from build123d import *

# Parameters (mm, degrees)
F0_R     = 1.778
F1_DEPTH = 6.7564
F3_R     = 1.1684
F4_DEPTH = 3.175
F5_R     = 1.143
F6_DEPTH = 3.175


with BuildPart() as f1:
    # F0 (on Top) → F1 (new body)
    with BuildSketch(Plane.XY):
        Circle(F0_R)
    extrude(amount=F1_DEPTH)

    # F3 (on face) → F4 (cut)
    with BuildSketch(Plane.XY.offset(6.7564)):
        Circle(F3_R)
    extrude(amount=F4_DEPTH, mode=Mode.SUBTRACT)

    # F5 (on face) → F6 (join)
    with BuildSketch(Plane(origin=(0, 0, 0), x_dir=(1, 0, 0), z_dir=(0, 0, -1))):
        Circle(F5_R)
    extrude(amount=F6_DEPTH)


solid = f1.part
The model under review builds one solid part; all positions refer to its coordinate system, in mm. A direction names the side the tool comes from. Round coordinates to 2 decimals unless told otherwise and drop trailing zeros. Loops run counter-clockwise (first coordinate to the right, second up) from the corner with the lowest first, then second, coordinate; pieces in that order, holes last. Notation, with made-up numbers: (-10.5, 56.25) -> (7.5, 56.25) arc R30 cw to (7.5, 83.25) -> close; hole circle Ø9 at (-37.5, -36.75). An arc over 180 degrees is marked (long way). Return JSON: item names as keys, results as strings.
(1) For pin 1 (1 mm diameter, centred on x = 0.5, z = -1, fed in from +Y); pin 2 (1.5 mm diameter, centred on y = 1, z = 3.5, fed in from -X); pin 3 (1 mm diameter, centred on y = -1.5, z = 4, fed in from +X), all flat-tipped, find the tip position at first contact; note any pin that passes through.
Solved:
{"pin 1": "y = 1.14", "pin 2": "x = -1.76", "pin 3": "x = 1.47"}
(2) Add section D-D on z = -0.5. Write out the cut boundary in (x, y).
Solved:
{"outline": "circle Ø2.29 at (0, 0)"}
(3) For line 1 (Z direction, x = 1.3, y = -0.3); line 2 (X direction, y = 0.4, z = 4.75); line 3 (X direction, y = -1.35, z = 6), list the stretches that pass through material, from the lowest coordinate up.
Solved:
{"line 1": "0 to 6.76", "line 2": "-1.73 to 1.73", "line 3": "-1.16 to 1.16"}
(4) Add section A-A on y = 0. Write out the cut boundary in (x, z) (3 decimals).
Solved:
{"outline": "(-1.778, 0) -> (-1.143, 0) -> (-1.143, -3.175) -> (1.143, -3.175) -> (1.143, 0) -> (1.778, 0) -> (1.778, 6.756) -> (-1.778, 6.756) -> close"}
(5) For faces 1 (the flat face through (-1, 1, 0)), 2 (the flat face through (0, 0, 6.756)), list the 3-axis set-ups (+Z, -Z, +X, -X, +Y, -Y) from which the entire face can be reached by the end or side of a thin tool; tool diameter is ignored.
Solved:
{"face 1": "-Z", "face 2": "+Z, +X, -X, +Y, -Y"}
(6) Add section C-C on z = 3. Write out the cut boundary in (x, y).
Solved:
{"outline": "circle Ø3.56 at (0, 0)"}
